from build123d import *

# Parameters (mm, degrees)
F1_DEPTH = 30
F2_W     = 10
F2_H     = 2.5
F3_DEPTH = 10
F4_W     = 10
F4_H     = 5
F5_W     = 10
F5_H     = 5
F6_DEPTH = 2


with BuildPart() as f1:
    # F0 (on Top) → F1 (new body)
    with BuildSketch(Plane.XY):
        Polygon((-93.994949, 98.994949), (-103.994949, 98.994949), (-2, 0), (-16.142136, -14.142136), (-14.142136, -16.142136), (0, -2), (14.142136, -16.142136), (16.142136, -14.142136), (2, 0), (16.142136, 14.142136), (14.142136, 16.142136), (0, 2), align=None)
    extrude(amount=F1_DEPTH)

    # F2 (on face) → F3 (join)
    with BuildSketch(Plane(origin=(0, 98.994949, 0), x_dir=(-1, 0, 0), z_dir=(0, 1, 0))):
        with Locations((98.994949, 1.25)):
            Rectangle(F2_W, F2_H)
        with Locations((98.994949, 28.75)):
            Rectangle(F2_W, F2_H)
    extrude(amount=F3_DEPTH)

    # F4 (on face) + F5 (on face) → F6 (join)
    with BuildSketch(Plane(origin=(0, 108.994949, 0), x_dir=(-1, 0, 0), z_dir=(0, 1, 0))):
        with Locations((98.994949, 2.5)):
            Rectangle(F4_W, F4_H)
    with BuildSketch(Plane(origin=(0, 108.994949, 0), x_dir=(-1, 0, 0), z_dir=(0, 1, 0))):
        with Locations((98.994949, 27.5)):
            Rectangle(F5_W, F5_H)
    extrude(amount=F6_DEPTH)


solid = f1.part
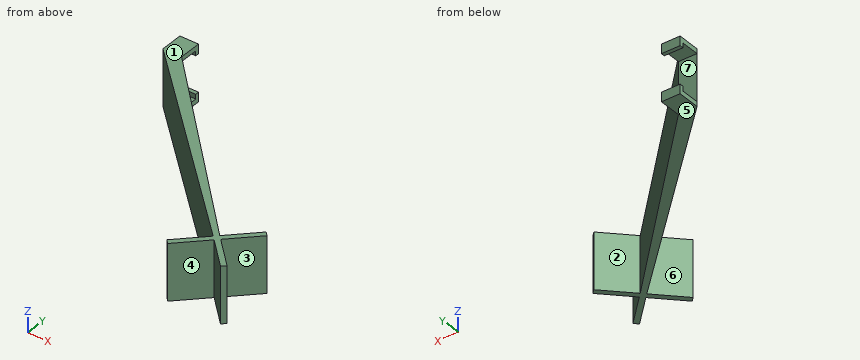
Design review of the part built by this model. Coordinates are the model's own, in mm. Face numbers are marked on the shaded views. A direction names the side the tool comes from. Give positions to 0.01 mm unless a question says otherwise; leave off trailing zeros. Loops run counter-clockwise (first coordinate to the right, second up) from the corner with the lowest first, then second, coordinate; pieces in that order, holes last. Notation, with made-up numbers: M 67.5,35.5 L 110.5,35.5 A15 cw 110.5,58.5 Z; hole C 24.5,-13 d7. An arc over 180 degrees is marked long. Write item = value, one per line.
Q1. We need section B-B (z = 8.75). Give the boundary of the cut face in (x, y).
Output values:
outline = M -103.99,98.99 L -2,0 L -16.14,-14.14 L -14.14,-16.14 L 0,-2 L 14.14,-16.14 L 16.14,-14.14 L 2,0 L 16.14,14.14 L 14.14,16.14 L 0,2 L -93.99,98.99 Z
Q2. We need section A-A (x = 6). Give the boundary of the cut face in (y, z), plus the area to 3 significant figures.
Output values:
outline = M -8,0 L -4,0 L -4,30 L -8,30 Z; M 4,0 L 8,0 L 8,30 L 4,30 Z
area = 240 mm^2
Q3. To check wall thickness, follow line 1 (Y direction, x = -15, z = 10.75); line 2 (X direction, y = -8, z = 26); line 3 (Y direction, x = -9.5, z = 13). State the ranges of each line that lie inside material, in increasing order. Write a range as [from, to].
Output values:
line_1 = [-15.28, -13], [12.62, 17.48]
line_2 = [-10, -6], [6, 10]
line_3 = [-11.5, -7.5], [7.28, 11.8]
Q4. Insertion check: pin 1 (0.8 mm diameter, centred on x = -100.5, z = 26, fed in from -Y); pin 2 (4 mm diameter, centred on x = -8, z = 20, fed in from -Y); pin 3 (2.5 mm diameter, centred on y = 103.5, z = 28, fed in from +X). Each pin has a flat end and moves straight along its axis. Give the tip position at first contact, or say it passes through.
Output values:
pin_1 = 95.21
pin_2 = -12
pin_3 = -93.99
Q5. We need section C-C (x = -97). Give the boundary of the cut face in (y, z), plus the area to 3 significant figures.
Output values:
outline = M 92.21,0 L 110.99,0 L 110.99,5 L 108.99,5 L 108.99,2.5 L 98.99,2.5 L 98.99,27.5 L 108.99,27.5 L 108.99,25 L 110.99,25 L 110.99,30 L 92.21,30 Z
area = 274 mm^2
Q6. Draft analysis for pull direction Y (two halves, no side actions). For the marked faces 1, 2 and 3, state which applies: +Y half, -Y half, draft (parallel to the pull), parting line (faces both ways), or undercut.
Output values:
face_1 = draft
face_2 = +Y half
face_3 = undercut
Q7. For the marked faces 4, 5, 6 and 7, list the 3-axis set-ups (+Z, -Z, +X, -X, +Y, -Y) from which the entire face can be reached by the end or side of a thin tool; tool diameter is ignored.
Output values:
face_4 = +Z, -Z, -Y
face_5 = -Z, +X, -X, +Y, -Y
face_6 = +Z, -Z, -X
face_7 = +X, -X
Q8. We need section D-D (y = 67). Give the boundary of the cut face in (x, z), plus the area to 3 significant figures.
Output values:
outline = M -71.03,0 L -62.99,0 L -62.99,30 L -71.03,30 Z
area = 241 mm^2
